Could you check a few things on this model? Use its own coordinates, in mm. A direction names the side the tool comes from. Give positions to 0.01 mm unless a question says otherwise; leave off trailing zeros. Write each loop counter-clockwise with the first axis right and the second up, starting at its lowest first coordinate (ties: lowest second). Pieces come first, ordered by that corner, then holes. Notation, with made-up numbers: M 44,35 L 70,35 A24 ccw 70,61 Z; hole C -2,1.5 d8. An arc over 180 degrees is marked long. Answer as CSV lines item,"result". Start each with the question number.
from build123d import *

# Parameters (mm, degrees)
F0_W     = 102
F0_H     = 50
F0_R     = 2.75
F1_DEPTH = 5
F2_W     = 102
F2_H     = 15
F3_DEPTH = 15
F4_SIZE  = 13
F5_R     = 15
F6_R     = 5.25
F7_DEPTH = 5


with BuildPart() as f1:
    # F0 (on Top) → F1 (new body)
    with BuildSketch(Plane.XY):
        with Locations((35.2871024236, -14.6758168936)):
            Rectangle(F0_W, F0_H)
        with Locations((19.2871024236, -30.6758168936)):
            Circle(F0_R, mode=Mode.SUBTRACT)
        with Locations((51.2871024236, -30.6758168936)):
            Circle(F0_R, mode=Mode.SUBTRACT)
        with Locations((19.2871024236, 1.3241831064)):
            Circle(F0_R, mode=Mode.SUBTRACT)
        with Locations((51.2871024236, 1.3241831064)):
            Circle(F0_R, mode=Mode.SUBTRACT)
    extrude(amount=F1_DEPTH)

    # F2 (on face) → F3 (join)
    with BuildSketch(Plane.XY.offset(5)):
        with Locations((35.2871024236, -12.1758168936)):
            Rectangle(F2_W, F2_H)
    extrude(amount=F3_DEPTH)

    # F4
    f4_edges = [f1.edges().sort_by_distance(p)[0] for p in [
        (35.287102, -19.675817, 20),
    ]]
    chamfer(f4_edges, length=F4_SIZE)

    # F5
    f5_edges = [f1.edges().sort_by_distance(p)[0] for p in [
        (86.287102, 10.324183, 2.5),
        (-15.712898, 10.324183, 2.5),
        (86.287102, -39.675817, 2.5),
        (-15.712898, -39.675817, 2.5),
    ]]
    fillet(f5_edges, radius=F5_R)

    # F6 (on face) → F7 (cut)
    with BuildSketch(Plane(origin=(0, -13.3379084468, 13.3379084468), x_dir=(1, 0, 0), z_dir=(0, -0.7071067812, 0.7071067812))):
        with Locations((0.2871024236, 0.2292320729)):
            Circle(F6_R)
        with Locations((70.2871024236, 0.2292320729)):
            Circle(F6_R)
    extrude(amount=-F7_DEPTH, mode=Mode.SUBTRACT)


solid = f1.part
1. Please list where these lines run through material, in increasing order: line 1 (X direction, y = -29, z = 4.75); line 2 (Z direction, x = -3.5, y = 4); line 3 (X direction, y = -7, z = 12.75).
2. Thinking about a two-plate mould opening in Y: for faces 5 (the flat face through (35, 10.324, 2)), 6 (the flat face through (86.287, -13, 8)), 7 (the cylindrical face through (21.827, 0.271, 2.465)), 8 (the cylindrical face through (53.91, -29.85, 2.46)), which applies, pulls with the +Y half, pulls with the -Y half, needs draft (parallel to the pull), parting line crosses it, or undercut?
3. Imagine slicing it at C-C, the plane z = 18.5. Please give me the cut outline in (x, y), plus the area to 3 significant figures.
4. Imagine slicing it at A-A, the plane x = 57. Please give me the cut outline in (y, z).
5. On a 3-axis mill with a long thin cutter (end or side, diameter ignored), from which of +Z, -Z, +X, -X, +Y, -Y can I reach the whole of each face in a straight line? I mean faces 1 (the flat face through (70.214, -9.588, 10.016)), 2 (the flat face through (35, -6, 20)), 3 (the flat face through (35, -4.676, 12)), 4 (the flat face through (35, -30, 5)). Say none if no direction works.
6. Imagine slicing it at D-D, the plane y = -3. Please give me the cut outline in (x, z), plus the area to 3 significant figures.
7. Will these pins go through, and if not, where does the flat tip stop? P1, Ø1, axis at x = 36.5, y = -11.5, coming from the +Z side; P2, Ø0.6, axis at x = 59, z = 6, coming from the -Y side; P3, Ø10, axis at x = 4, z = 14, coming from the +Y side; P4, Ø10, axis at x = 19.5, y = -21.5, coming from the -Z side.
8. Imagine slicing it at B-B, the plane x = 73.5. Please give me the cut outline in (y, z), plus the area to 3 significant figures.
Solutions:
1,line 1,"-15.08 to 17.11, 21.47 to 49.11, 53.47 to 85.65"
1,line 2,"0 to 5"
1,line 3,"-15.71 to -3.3, 3.87 to 66.7, 73.87 to 86.29"
2,face 5,"pulls with the +Y half"
2,face 6,"needs draft"
2,face 7,"undercut"
2,face 8,"undercut"
3,outline,"M -15.71,-8.18 L 86.29,-8.18 L 86.29,-4.68 L -15.71,-4.68 Z"
3,area,"357 mm²"
4,outline,"M -39.68,0 L 10.32,0 L 10.32,5 L -4.68,5 L -4.68,20 L -6.68,20 L -19.68,7 L -19.68,5 L -39.68,5 Z"
5,face 1,"none"
5,face 2,"+Z, +X, -X, +Y, -Y"
5,face 3,"+Z, +X, -X, +Y"
5,face 4,"+Z, +X, -X, -Y"
6,outline,"M -15.62,0 L 86.19,0 L 86.19,5 L -15.62,5 Z"
6,area,"509 mm²"
7,P1,"z = 15.68"
7,P2,"y = -19.68"
7,P3,"y = -4.68"
7,P4,"z = 0"
8,outline,"M -39.51,0 L 10.16,0 L 10.16,5 L -4.68,5 L -4.68,20 L -6.68,20 L -10.24,16.44 L -6.7,12.9 L -12.58,7.03 L -16.11,10.56 L -19.68,7 L -19.68,5 L -39.51,5 Z"
8,area,"347 mm²"
